Here's how the part is built. I have some questions about the finished solid (model axes, mm). Face numbers are marked on the shaded views. A direction names the side the tool comes from. Round coordinates to 2 decimals unless told otherwise and drop trailing zeros. Order: outer loops, then holes, each group sorted by start corner. A loop starts at its lowest first (then second) coordinate and runs counter-clockwise, first axis right, second up. Notation, with made-up numbers: (-7.5, -3) -> (2.5, -3) arc R23 cw to (2.5, 7) -> close; hole circle Ø2 at (47.25, 78). An arc over 180 degrees is marked (long way). Use a Markdown table: item, result. Add a question column.
(1) If I drill on probe 1 along Z at (x, y) = (0, 1.45); probe 2 along Z at (x, y) = (-28.5, 39); probe 3 along Y at (x, z) = (54, 22.25), over which ranges is the centre line in solid material (lowest first)?
(2) I want a section at A-A, the plane x = 0. Please give me the cut outline in (y, z).
(3) I want a section at D-D, the plane x = 49.5. Please give me the cut outline in (y, z), then the cut area to 3 significant figures.
(4) I want a section at B-B, the plane z = 6. Please give me the cut outline in (x, y), then the cut area to 3 significant figures.
(5) I'm going to push flat-ended pins straight in: P1, Ø8, axis at x = -8.5, z = 6, coming from the +Y side; P2, Ø8, axis at y = 42, z = 7.5, coming from the -X side; P3, Ø4, axis at x = 22, z = 4, coming from the +Y side; P4, Ø6, axis at y = 8, z = 4, coming from the -X side. Where does each tip first touch, or does it pass through?
(6) I want a section at C-C, the plane y = 11.5. Please give me the cut outline in (x, z), then the cut area to 3 significant figures.
(7) Thinking about a two-plate mould opening in X: for the marked faces 1, 2, 3 and 4, which applies, pulls with the +X half, pulls with the -X half, needs draft (parallel to the pull), parting line crosses it, or undercut?
(8) On a 3-axis mill with a long thin cutter (end or side, diameter ignored), from which of +Z, -Z, +X, -X, +Y, -Y can I reach the whole of each face in a straight line? I mean the marked faces 5 and 6. Say none if no direction works.
from build123d import *

# Parameters (mm, degrees)
F1_DEPTH = 25
F2_T     = -2.3
F4_D     = 5.5
F4_DEPTH = 12
F4_TIP   = 1.6523667023


with BuildPart() as f1:
    # F0 (on Top) → F1 (new body)
    with BuildSketch(Plane.XY):
        with BuildLine():
            ThreePointArc((-40.594752878, 26.4406520873), (-55.3794762118, 17.3284085078), (-54.2187498458, 0))
            Line((-54.2187498458, 0), (65.7812501542, 0))
            ThreePointArc((65.7812501542, 0), (63.8571902729, 23.0404540262), (40.9879274666, 26.4406520873))
            ThreePointArc((40.9879274666, 26.4406520873), (18.0492419713, 53.7154868807), (-13.8592263684, 37.8425680101))
            ThreePointArc((-13.8592263684, 37.8425680101), (-30.9125269305, 40.7835594412), (-40.594752878, 26.4406520873))
        make_face()
    extrude(amount=F1_DEPTH)

    # F2
    f2_openings = [f1.faces().sort_by_distance(p)[0] for p in [
        (5.721162, 21.020998, 25),
    ]]
    offset(amount=F2_T, openings=f2_openings, kind=Kind.INTERSECTION)

    # F4
    with Locations(Plane.XZ):
        with Locations((0, 6)):
            Hole(F4_D / 2, depth=F4_DEPTH)
            with Locations((0, 0, -(F4_DEPTH + F4_TIP / 2))):  # 118° drill point
                Cone(0, F4_D / 2, F4_TIP, mode=Mode.SUBTRACT)


solid = f1.part
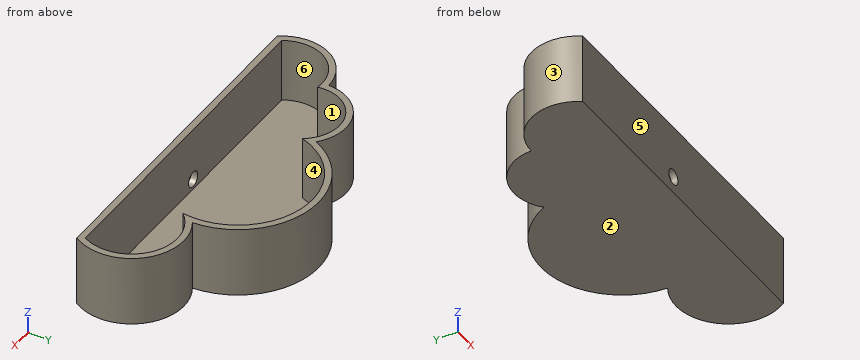
Taken from the geometry:
| question | item | result |
|---|---|---|
| 1 | probe 1 | z = 0 to 3.25, 8.75 to 25 |
| 1 | probe 2 | z = 0 to 2.3 |
| 1 | probe 3 | y = 0 to 2.3, 26.19 to 28.55 |
| 2 | outline | (0, 0) -> (51.62, 0) -> (51.62, 25) -> (49.05, 25) -> (49.05, 2.3) -> (2.3, 2.3) -> (2.3, 3.25) -> (0, 3.25) -> close; (0, 8.75) -> (2.3, 8.75) -> (2.3, 25) -> (0, 25) -> close |
| 3 | outline | (0, 0) -> (28.91, 0) -> (28.91, 25) -> (26.6, 25) -> (26.6, 2.3) -> (2.3, 2.3) -> (2.3, 25) -> (0, 25) -> close |
| 3 | area | 171 mm2 |
| 4 | outline | (-54.22, 0) -> (-2.75, 0) -> (-2.75, 2.3) -> (-52.96, 2.3) arc R14.51 cw to (-38.12, 23.96) arc R13.64 cw to (-13.13, 33.41) arc R26.52 cw to (38.4, 21.49) arc R16.32 cw to (64.49, 2.3) -> (2.75, 2.3) -> (2.75, 0) -> (65.78, 0) arc R18.62 ccw to (40.99, 26.44) arc R28.82 ccw to (-13.86, 37.84) arc R15.94 ccw to (-40.59, 26.44) arc R16.81 ccw to start |
| 4 | area | 715 mm2 |
| 5 | P1 | stops at y = 49 |
| 5 | P2 | stops at x = -35.29 |
| 5 | P3 | stops at y = 53.24 |
| 5 | P4 | stops at x = -57.25 |
| 6 | outline | (-57.14, 0) -> (68.86, 0) -> (68.86, 25) -> (66.55, 25) -> (66.55, 2.3) -> (-54.83, 2.3) -> (-54.83, 25) -> (-57.14, 25) -> close |
| 6 | area | 395 mm2 |
| 7 | face 1 | undercut |
| 7 | face 2 | needs draft |
| 7 | face 3 | pulls with the -X half |
| 7 | face 4 | undercut |
| 8 | face 5 | +Z, -Z, +X, -X, -Y |
| 8 | face 6 | +Z |
